Autodesk Inventor part; units mm, degrees
ref_plane "YZ Plane" through (0, 0, 0) normal (1, 0, 0) x (0, 1, 0)
ref_plane "XZ Plane" through (0, 0, 0) normal (0, 1, 0) x (-1, 0, 0)
ref_plane "XY Plane" through (0, 0, 0) normal (0, 0, 1) x (1, 0, 0)
sketch "Sketch1" plane through (0, 0, 0) normal (0, 1, 0) x (-1, 0, 0)
  circle A0 centre (-20.6375, 35.7452) radius 2
  circle A1 centre (20.6375, 35.7452) radius 2
  line L0 (0, -10) -> (-10, -10)
  line L1 (-10, -10) -> (-10, 10)
  line L2 (-10, 10) -> (10, 10)
  line L3 (10, 10) -> (10, -10)
  line L4 (10, -10) -> (0, -10)
  arc A2 (23.6974, 27.5118) -> (-23.6974, 27.5118) centre (0, 0) ccw
  arc A3 (32.696, 32.7072) -> (-32.696, 32.7072) centre (0, 0) ccw
  line L5 (20.6375, 35.7452) -> (29.2978, 40.7452) construction
  line L6 (32.696, 32.7072) -> (23.6974, 27.5118)
  arc A4 (32.696, 32.7072) -> (-32.696, 32.7072) centre (0, 0) ccw
  line L7 (0, -10) -> (0, 10)
  line L8 (-32.696, 32.7072) -> (-23.6974, 27.5118)
  arc A5 (28.2185, 30.1221) -> (-28.2185, 30.1221) centre (0, 0) ccw
  dimension "d11" = 10
  dimension "d12" = 20
  dimension "d13" = 20
  dimension "d14" = 20
extrude "Extrusion11" add sketch "Sketch1" along normal blind 3 contours A0 A5 A1 L6 A2 L8 | A0 A5 L8 A3 L6 A1
sketch "Sketch6" plane through (0, 3, 0) normal (0, 1, 0) x (1, 0, 0)
  point P0 (0, 0)
sketch "Sketch7" plane through (0, 3, 0) normal (0, 1, 0) x (1, 0, 0)
  arc A0 (-10, -34.9065) -> (10, -34.9065) centre (0, 0) ccw
  arc A1 (-32.696, -32.7072) -> (32.696, -32.7072) centre (0, 0) ccw
  arc A2 (-23.6974, -27.5118) -> (23.6974, -27.5118) centre (0, 0) ccw
  line L0 (0, 0) -> (-10, 0)
  line L1 (10, -34.9065) -> (10, -45.1529)
  line L2 (-10, -34.9065) -> (-10, -45.1529)
  line L3 (-10, 0) -> (40, 0) construction
  arc A3 (-10, -45.1529) -> (10, -45.1529) centre (0, 0) ccw
extrude "Extrusion12" add sketch "Sketch7" along normal blind 28
sketch "Sketch8" plane through (0, 31, 0) normal (0, 1, 0) x (1, 0, 0)
  arc A0 (-10, -34.9065) -> (10, -34.9065) centre (0, 0) ccw
  arc A1 (-10, -45.1529) -> (10, -45.1529) centre (0, 0) ccw
  line L0 (10, -34.9065) -> (10, -45.1529)
  line L1 (10, -34.9065) -> (10, -45.1529)
  arc A2 (-23.6974, -27.5118) -> (23.6974, -27.5118) centre (0, 0) ccw
  line L2 (-10, -34.9065) -> (-10, -45.1529)
  arc A3 (-32.696, -32.7072) -> (32.696, -32.7072) centre (0, 0) ccw
extrude "Extrusion13" add sketch "Sketch8" along normal blind 5
sketch "Sketch9" plane through (0, 36, 0) normal (0, 1, 0) x (1, 0, 0)
  line L0 (0, 0) -> (0, 10)
  line L1 (0, 10) -> (10, 10)
  line L2 (10, 10) -> (10, -10)
  line L3 (10, -10) -> (-10, -10)
  line L4 (-10, -10) -> (-10, 10)
  line L5 (-10, 10) -> (0, 10)
  dimension "d63" = 10
  dimension "d64" = 10
  dimension "d65" = 20
  dimension "d66" = 20
  dimension "d67" = 20
extrude "Extrusion14" add sketch "Sketch9" against normal blind 5
sketch "Sketch10" plane through (10, 36, -10) normal (0, 0, -1) x (-1, 0, 0)
  line L0 (0, 0) -> (20, 0)
  line L1 (20, 0) -> (20, -3)
  line L2 (20, -33) -> (20, 0)
  line L3 (20, -3) -> (0, -3)
  line L4 (20, -5) -> (0, -5)
  line L5 (0, -33) -> (0, 0)
  line L6 (0, -3) -> (0, 0)
  line L7 (0, 0) -> (20, 0)
  point P0 (10, -36)
  dimension "d70" = 3
  dimension "d71" = 20
  dimension "d72" = 90
extrude "Extrusion15" add sketch "Sketch10" against normal blind 50 contours L0 L1 L3 L5
properties part number "Corona_Cam_Setup_Tool._v2ipt"
CAD build for the part. Positions are in the model's coordinates, mm. A direction names the side the tool comes from. Give positions to 0.01 mm unless a question says otherwise; leave off trailing zeros. Loops run counter-clockwise (first coordinate to the right, second up) from the corner with the lowest first, then second, coordinate; pieces in that order, holes last. Notation, with made-up numbers: M -15,-9 L 10,-9 A21 ccw 10,21 Z; hole C -15,43 d10. An arc over 180 degrees is marked long. Use one line per item in the form item = value.
Item 1: Flat gauge pins, fed straight in: pin 1 (12 mm diameter, centred on x = -17.5, y = 10, fed in from -Z); pin 2 (1.5 mm diameter, centred on x = 23, z = 34, fed in from +Y); pin 3 (3 mm diameter, centred on x = 9, y = 6.5, fed in from -Z); pin 4 (4 mm diameter, centred on y = 15, z = 33.5, fed in from +X). Where does each tip first touch, or does it go through?
Determined:
pin_1 = through
pin_2 = 3
pin_3 = 34.91
pin_4 = 10
Item 2: Slice it at C-C (y = 28). List the corners of the cut face in (x, z).
Determined:
outline = M -10,34.91 A36.31 cw 10,34.91 L 10,45.15 A46.25 ccw -10,45.15 Z
Item 3: Which spindle directions (+Z, -Z, +X, -X, +Y, -Y) get a long thin tool onto all of the face, cutting with end or side? Do faces 4 (the face through (10, 26, 36)), 5 (the face through (0, 32, 10)), 6 (the face through (0, 31, 0)), 7 (the face through (-19, 3, 34)). Say none if no direction does.
Determined:
face_4 = +Z, -Z, +X, +Y
face_5 = +X, -X, -Y
face_6 = -Z, +X, -X, -Y
face_7 = +Z, -Z, -X, +Y
Item 4: Two-plate mould, pull along X, no slides. Class faces 1 (the face through (0.36, 1.48, 36.31)), 2 (the face through (-28.26, 1.479, 30.146)), 3 (the face through (0, 34, -10)): pulls with the +X half, pulls with the -X half, needs draft (parallel to the pull), parting line crosses it, or undercut.
Determined:
face_1 = undercut
face_2 = pulls with the -X half
face_3 = needs draft
Item 5: Slice it at A-A (z = 28.5). List the corners of the cut face in (x, y), plus the area to 3 significant figures.
Determined:
outline = M -25.41,0 L -22.5,0 L -22.5,3 L -25.41,3 Z; M -10,33 L 10,33 L 10,36 L -10,36 Z; M 22.5,0 L 25.41,0 L 25.41,3 L 22.5,3 Z
area = 77.5 mm2
Item 6: Slice it at D-D (z = 9). List the corners of the cut face in (x, y).
Determined:
outline = M -10,31 L 10,31 L 10,36 L -10,36 Z
Item 7: Drill centre lines: probe 1 along X at (y, z) = (13.5, 39.5); probe 2 along Z at (x, y) = (1, 18); probe 3 along Y at (x, z) = (13.5, 39.5). Where is each one in solid material? Low to high. Write a range as from..to.
Determined:
probe_1 = -10..10
probe_2 = 36.3..46.24
probe_3 = 0..3
Item 8: Slice it at B-B (x = 4). List the corners of the cut face in (y, z), plus the area to 3 significant figures.
Determined:
outline = M 0,36.09 L 33,36.09 L 33,10 L 31,10 L 31,-10 L 36,-10 L 36,46.07 L 0,46.07 Z
area = 538 mm2
